Here's how the part is built. I have some questions about the finished solid (model axes, mm). Give positions to 0.01 mm unless a question says otherwise; leave off trailing zeros. Loops run counter-clockwise (first coordinate to the right, second up) from the corner with the lowest first, then second, coordinate; pieces in that order, holes last.
Q1. I need wall thicknesses on probe 1 along Y at (x, z) = (0.65, -242); probe 2 along Y at (x, z) = (-0.6, 258); probe 3 along Z at (x, y) = (1.1, 5). Which ranges of each line are inside material? Lowest first, please.
Q2. Thinking about a two-plate mould opening in Y: for faces 1 (the face through (0.022, -2.681, 243.534)), 2 (the face through (-0.022, -0.495, 272.495)), 3 (the face through (1.588, 0, 4)), which applies, pulls with the +Y half, pulls with the -Y half, needs draft (parallel to the pull), parting line crosses it, or undercut?
Q3. I'm going to push flat-ended pins straight in: P1, Ø5, axis at y = 8, z = -258, coming from the -X side; P2, Ø1, axis at x = 0, y = 16, coming from the -Z side. Where does each tip first touch, or does it pass through?
Q4. Suppose I cut it at B-B (x = 0). Count the separate pieces of the cut face and the enclosed holes in it, and give its area (3 significant figures).
Q5. Suppose I cut it at A-A (y = 0). List the corners of the cut face in (x, z) for me.
Autodesk Inventor part; units mm, degrees
ref_plane "YZ Plane" through (0, 0, 0) normal (1, 0, 0) x (0, 1, 0)
ref_plane "XZ Plane" through (0, 0, 0) normal (0, 1, 0) x (-1, 0, 0)
ref_plane "XY Plane" through (0, 0, 0) normal (0, 0, 1) x (1, 0, 0)
sketch "Sketch1" plane through (0, 0, 0) normal (1, 0, 0) x (0, 1, 0)
  line L0 (-22.5, 250) -> (22.5, 250) construction
  line L1 (22.5, 250) -> (22.5, -250)
  line L2 (22.5, -250) -> (-22.5, -250) construction
  line L3 (-22.5, -250) -> (-22.5, 250)
  line L4 (-22.5, 250) -> (22.5, -250) construction
  line L5 (22.5, 250) -> (-22.5, -250) construction
  arc A0 (-22.5, -250) -> (22.5, -250) centre (0, -250) ccw
  arc A1 (22.5, 250) -> (-22.5, 250) centre (0, 250) ccw
  point P0 (0, 0)
  dimension "d0" = 45
  dimension "d1" = 500
extrude "Extrusion2" add sketch "Sketch1" along normal mid plane 3.175
sketch "Sketch3" plane through (1.5875, 0, 0) normal (1, 0, 0) x (0, 0, -1)
  line L0 (250, 22.5) -> (-250, 22.5) construction
  arc A0 (-250, 22.5) -> (-250, -22.5) centre (-250, 0) ccw construction
  line L1 (-250, -22.5) -> (250, -22.5) construction
  arc A1 (250, -22.5) -> (250, 22.5) centre (250, 0) ccw construction
  circle A2 centre (-250, 0) radius 7
  circle A3 centre (-258, 8) radius 2
  circle A4 centre (-258, -8) radius 2
  circle A5 centre (-242, -8) radius 2
  circle A6 centre (-242, 8) radius 2
  line L2 (0, 22.5) -> (0, -22.5) construction
  circle A7 centre (250, 0) radius 7
  circle A8 centre (258, 8) radius 2
  circle A9 centre (258, -8) radius 2
  circle A10 centre (242, -8) radius 2
  circle A11 centre (242, 8) radius 2
  point P0 (0, 0)
  dimension "d14" = 14
  dimension "d15" = 4
  dimension "d16" = 8
  dimension "d17" = 8
  dimension "d20" = 360
extrude "Extrusion3" cut sketch "Sketch3" against normal through all
properties part number "ArmBarStage1"
Solutions:
1. probe 1: y = -22.5 to -10, -6 to 6, 10 to 22.5
1. probe 2: y = -21.03 to -10, -6 to 6, 10 to 21.03
1. probe 3: z = -271.94 to -254.9, -245.1 to 245.1, 254.9 to 271.94
2. face 1: undercut
2. face 2: parting line crosses it
2. face 3: needs draft
3. P1: stops at x = -1.59
3. P2: stops at z = -266.31
4. separate pieces: 1
4. enclosed holes: 10
4. area: 23,700 mm2
5. outline: (-1.59, -272.5) - (1.59, -272.5) - (1.59, -257) - (-1.59, -257) - close; (-1.59, -243) - (1.59, -243) - (1.59, 243) - (-1.59, 243) - close; (-1.59, 257) - (1.59, 257) - (1.59, 272.5) - (-1.59, 272.5) - close
